```python
from build123d import *

# Parameters (mm, degrees)
SKETCH_1_R          = 1.6
EXTRUDE_1_DEPTH     = 12
CUT_EXTRUDE_1_DEPTH = 21
CUT_EXTRUDE_6_DEPTH = 21
SKETCH_12_R         = 1.6
EXTRUDE_11_DEPTH    = 5
SKETCH_13_R         = 1.6
EXTRUDE_12_DEPTH    = 5
SKETCH_14_W         = 2.04
SKETCH_14_H         = 20
CUT_EXTRUDE_7_DEPTH = 21
SKETCH_15_W         = 6
SKETCH_15_H         = 6
EXTRUDE_13_DEPTH    = 68
SKETCH_17_R         = 1.6
CUT_EXTRUDE_8_DEPTH = 18
CHAMFER_1_SIZE      = 0.5


with BuildPart() as part:
    # 草圖1 → 填料-伸長1 (new body)
    with BuildSketch(Plane.XY):
        with BuildLine():
            Line((-10, 0), (-10, -30.276417548))
            Line((-10, -30.276417548), (10, -30.276417548))
            Line((10, -30.276417548), (10, 0))
            ThreePointArc((10, 0), (0, 10), (-10, 0))
        make_face()
        Circle(SKETCH_1_R, mode=Mode.SUBTRACT)
    extrude(amount=EXTRUDE_1_DEPTH)

    # 草圖2 → 除料-伸長1 (cut, through all)
    with BuildSketch(Plane(origin=(10, 0, 0), x_dir=(0, 0, -1), z_dir=(1, 0, 0))):
        Polygon((-9, 0), (-6, 0), (-3, 0), (-3, 15.780779257), (-9, 15.780779257), align=None)
        Polygon((-3, 0), (-6, 0), (-9, 0), (-8.60053373, -20), (-3, -20), align=None)
    extrude(amount=-CUT_EXTRUDE_1_DEPTH, mode=Mode.SUBTRACT)

    # 草圖11 → 除料-伸長6 (cut, through all)
    with BuildSketch(Plane(origin=(10, 0, 0), x_dir=(0, 0, -1), z_dir=(1, 0, 0))):
        Polygon((-9, 0), (-9, -20), (-8.60053373, -20), align=None)
    extrude(amount=-CUT_EXTRUDE_6_DEPTH, mode=Mode.SUBTRACT)

    # 草圖12 → 填料-伸長11 (add)
    with BuildSketch(Plane.XY.offset(12)):
        with BuildLine():
            ThreePointArc((10, 0), (0, 10), (-10, 0))
            ThreePointArc((-10, 0), (0, -10), (10, 0))
        make_face()
        Circle(SKETCH_12_R, mode=Mode.SUBTRACT)
        with BuildLine():
            ThreePointArc((10, 0), (0, -10), (-10, 0))
            Line((-10, 0), (-10, -30.276417548))
            Line((-10, -30.276417548), (10, -30.276417548))
            Line((10, -30.276417548), (10, 0))
        make_face()
    extrude(amount=EXTRUDE_11_DEPTH)

    # 草圖13 → 填料-伸長12 (add)
    with BuildSketch(Plane(origin=(0, 0, 0), x_dir=(-1, 0, 0), z_dir=(0, 0, -1))):
        with BuildLine():
            ThreePointArc((10, 0), (0, 10), (-10, 0))
            ThreePointArc((-10, 0), (0, -10), (10, 0))
        make_face()
        Circle(SKETCH_13_R, mode=Mode.SUBTRACT)
        with BuildLine():
            ThreePointArc((10, 0), (0, -10), (-10, 0))
            Line((-10, 0), (-10, -30.276417548))
            Line((-10, -30.276417548), (10, -30.276417548))
            Line((10, -30.276417548), (10, 0))
        make_face()
    extrude(amount=EXTRUDE_12_DEPTH)

    # 草圖14 → 除料-伸長7 (cut, through all)
    with BuildSketch(Plane.ZY.offset(10)):
        Polygon((3, 0), (3, -20), (9, -20), (9, 0), (11.04, 0), (11.04, 10), (3, 10), (0.96, 10), (0.96, 0), align=None)
        with Locations((1.98, -10)):
            Rectangle(SKETCH_14_W, SKETCH_14_H)
        with Locations((10.02, -10)):
            Rectangle(SKETCH_14_W, SKETCH_14_H)
    extrude(amount=-CUT_EXTRUDE_7_DEPTH, mode=Mode.SUBTRACT)

    # 草圖15 → 填料-伸長13 (add)
    with BuildSketch(Plane.XZ.offset(30.276417548)):
        with Locations((3, 9)):
            Rectangle(SKETCH_15_W, SKETCH_15_H)
        with Locations((-3, 9)):
            Rectangle(SKETCH_15_W, SKETCH_15_H)
        with Locations((3, 3)):
            Rectangle(SKETCH_15_W, SKETCH_15_H)
        with Locations((-3, 3)):
            Rectangle(SKETCH_15_W, SKETCH_15_H)
    extrude(amount=EXTRUDE_13_DEPTH)

    # 草圖17 → 除料-伸長8 (cut, through all)
    with BuildSketch(Plane(origin=(0, 0, 0), x_dir=(-1, 0, 0), z_dir=(0, 0, -1))):
        with Locations((0, -93.276417548)):
            Circle(SKETCH_17_R)
    extrude(amount=-CUT_EXTRUDE_8_DEPTH, mode=Mode.SUBTRACT)

    # 導角1
    chamfer_1_edges = [part.edges().sort_by_distance(p)[0] for p in [
        (10, -30.276417548, 6),
        (-10, -30.276417548, 6),
        (0, -30.276417548, 17),
        (0, 10, -5),
        (10, -15.138208774, -5),
        (0, -30.276417548, -5),
        (-10, -15.138208774, -5),
    ]]
    chamfer(chamfer_1_edges, length=CHAMFER_1_SIZE)


solid = part.part
```
Build history of the part. All positions in model axes, mm. A direction names the side the tool comes from. Round coordinates to 2 decimals unless told otherwise and drop trailing zeros. Write each loop counter-clockwise with the first axis right and the second up, starting at its lowest first coordinate (ties: lowest second). Pieces come first, ordered by that corner, then holes.
1) Band-saw the part on B-B, the plane x = 0. List the corners of the cut face in (y, z).
2) Pin check, flat tips, straight feed: pin 1 (10 mm diameter, centred on y = -69.5, z = 0.5, fed in from -X); pin 2 (12 mm diameter, centred on y = -74, z = 0.5, fed in from +X); pin 3 (12 mm diameter, centred on x = 7.5, y = -87, fed in from +Z). Stop position of each tip, or through.
3) Band-saw the part on A-A, the plane y = -17.5. List the corners of the cut face in (x, z).
4) 3-axis set-ups, long thin cutter, end or side, ignore diameter. For faces 4 (the flat face through (-6, -64, 6)), 5 (the flat face through (0, -64, 12)), 6 (the flat face through (0, -64, 0)): which of +Z, -Z, +X, -X, +Y, -Y reach the whole face in a straight line?
5) Band-saw the part on D-D, the plane y = -68.5. List the corners of the cut face in (x, z), and give its area (3 significant figures).
6) Mould opens along Y. For faces 1 (the cylindrical face through (-1.27, -0.97, 13.98)), 2 (the flat face through (0, -98.276, 6)), 3 (the flat face through (0, -5, 11.04)) say: +Y half, -Y half, draft (parallel to the pull), parting line (faces both ways), or undercut.
7) Band-saw the part on C-C, the plane z = -3.5. List the corners of the cut face in (x, y), and give its area (3 significant figures).
8) Drill centre lines: probe 1 along Y at (x, z) = (0, 0.6); probe 2 along Y at (x, z) = (0, 10); probe 3 along Y at (x, z) = (0, 14.5). Where is each one in solid material? Low to high.
Ans:
1. outline: (-98.28, 0) - (-94.88, 0) - (-94.88, 12) - (-98.28, 12) - close; (-91.68, 0) - (-30.28, 0) - (-30.28, -4.5) - (-29.78, -5) - (-1.6, -5) - (-1.6, 0.96) - (-20, 0.96) - (-20, 11.04) - (-1.6, 11.04) - (-1.6, 17) - (-29.78, 17) - (-30.28, 16.5) - (-30.28, 12) - (-91.68, 12) - close; (1.6, -5) - (9.5, -5) - (10, -4.5) - (10, 0.96) - (1.6, 0.96) - close; (1.6, 11.04) - (10, 11.04) - (10, 17) - (1.6, 17) - close
2. pin 1: stops at x = -6
2. pin 2: stops at x = 6
2. pin 3: stops at z = 12
3. outline: (-10, -4.5) - (-9.5, -5) - (9.5, -5) - (10, -4.5) - (10, 0.96) - (-10, 0.96) - close; (-10, 11.04) - (10, 11.04) - (10, 17) - (-10, 17) - close
4. face 4: +Z, -Z, -X, -Y
4. face 5: +Z, +X, -X, -Y
4. face 6: -Z, +X, -X, -Y
5. outline: (-6, 0) - (6, 0) - (6, 12) - (-6, 12) - close
5. area: 144 mm2
6. face 1: undercut
6. face 2: -Y half
6. face 3: draft
7. outline: (-10, -29.78) - (-9.5, -30.28) - (9.5, -30.28) - (10, -29.78) - (10, 0) arc R10 ccw to (-10, 0) - close; hole circle Ø3.2 at (0, 0)
7. area: 754 mm2
8. probe 1: y = -98.28 to -94.88, -91.68 to -1.6, 1.6 to 10
8. probe 2: y = -98.28 to -94.88, -91.68 to -20
8. probe 3: y = -30.28 to -1.6, 1.6 to 10
